```python
from build123d import *

# Parameters (mm, degrees)
SKETCH1_R           = 14.1
BOSS_EXTRUDE1_DEPTH = 3
SKETCH2_R           = 14.1
SKETCH2_R_2         = 12.6
BOSS_EXTRUDE2_DEPTH = 50
CHAMFER1_SIZE       = 1


with BuildPart() as part:
    # Sketch1 → Boss-Extrude1 (new body)
    with BuildSketch(Plane(origin=(0, 0, 0), x_dir=(1, 0, 0), z_dir=(0, 1, 0))):
        with Locations(Location((0, 0, 0), (0, 0, 270))):
            Circle(SKETCH1_R)
    extrude(amount=BOSS_EXTRUDE1_DEPTH)

    # Sketch2 → Boss-Extrude2 (add)
    with BuildSketch(Plane(origin=(0, 3, 0), x_dir=(1, 0, 0), z_dir=(0, 1, 0))):
        with Locations(Location((0, 0, 0), (0, 0, 270))):
            Circle(SKETCH2_R)
        with Locations(Location((0, 0, 0), (0, 0, 270))):
            Circle(SKETCH2_R_2, mode=Mode.SUBTRACT)
    extrude(amount=BOSS_EXTRUDE2_DEPTH)

    # Chamfer1
    chamfer1_edges = [part.edges().sort_by_distance(p)[0] for p in [
        (0, 0, -14.1),
    ]]
    chamfer(chamfer1_edges, length=CHAMFER1_SIZE)


solid = part.part
```
Verification items for the finished model (mm, model axes). A direction names the side the tool comes from. Coordinates: 2 decimals unless noted, no trailing zeros. Loops run counter-clockwise (first coordinate to the right, second up) from the corner with the lowest first, then second, coordinate; pieces in that order, holes last. Notation, with made-up numbers: (18.5, -10) -> (40.5, -10) arc R20 cw to (40.5, 0) -> close; hole circle Ø11 at (-12.75, -0.5). An arc over 180 degrees is marked (long way). Put each result on its own line as item: value.
1. Tool access check on faces 4 (the face through (0, 0, 0)), 5 (the face through (0, 3, 0)). Record the directions out of +Z, -Z, +X, -X, +Y, -Y that give a thin tool (end or side, any length) a straight path to the whole face; none if there is none.
Result set:
face 4: +Z, -Z, +X, -X, -Y
face 5: +Y
2. Section check A-A, the plane z = 0. Record the boundary of the cut face in (x, y).
Result set:
outline: (-14.1, 1) -> (-13.1, 0) -> (13.1, 0) -> (14.1, 1) -> (14.1, 53) -> (12.6, 53) -> (12.6, 3) -> (-12.6, 3) -> (-12.6, 53) -> (-14.1, 53) -> close
3. Thickness scan on line 1 (X direction, y = 25.5, z = 0); line 2 (Y direction, x = 8.25, z = 0); line 3 (X direction, y = 29, z = 2.25). Record the ranges inside material, lowest first.
Result set:
line 1: x = -14.1 to -12.6, 12.6 to 14.1
line 2: y = 0 to 3
line 3: x = -13.92 to -12.4, 12.4 to 13.92
4. Section check C-C, the plane y = 18. Record the boundary of the cut face in (x, z).
Result set:
outline: circle Ø28.2 at (0, 0); hole circle Ø25.2 at (0, 0)
5. Section check B-B, the plane x = 0. Record the boundary of the cut face in (y, z).
Result set:
outline: (0, -13.1) -> (1, -14.1) -> (53, -14.1) -> (53, -12.6) -> (3, -12.6) -> (3, 12.6) -> (53, 12.6) -> (53, 14.1) -> (1, 14.1) -> (0, 13.1) -> close
6. Gauge pin test, flat ends, axial feed: P1, Ø5, axis at y = 40, z = 6, coming from the -X side; P2, Ø1, axis at x = -5, z = 9.5, coming from the +Y side; P3, Ø1.5, axis at y = 25.5, z = 11, coming from the -X side. Record the tip position at first contact, or that the pin passes through.
Result set:
P1: stops at x = -13.66
P2: stops at y = 3
P3: stops at x = -9.68
7. Mould release check, pull along Z, two halves, no side actions. Record for faces 1 (the face through (-7.667, 27.65, -9.999)), 2 (the face through (-5.4, 26.636, 13.025)), 3 (the face through (-7, 53, -11)): pulls with the +Z half, pulls with the -Z half, needs draft (parallel to the pull), parting line crosses it, or undercut.
Result set:
face 1: undercut
face 2: parting line crosses it
face 3: needs draft
